from build123d import *

# Parameters (mm, degrees)
BOSS_EXTRUDE1_DEPTH = 9.525
CUT_EXTRUDE11_DEPTH = 109.249530891
CUT_EXTRUDE12_DEPTH = 109.249530891
CUT_EXTRUDE1_DEPTH  = 164.459241155
FILLET25_R          = 0.79375
CUT_EXTRUDE8_DEPTH  = 7.112
FILLET31_R          = 0.79375
FILLET32_R          = 0.5
DELETEFACE2_START   = 2.413
DELETEFACE2_DEPTH   = 8.587
DELETEFACE2_2_DEPTH = 9.525
DELETEFACE3_START   = 2.413
DELETEFACE3_DEPTH   = 7.112
SKETCH42_R          = 2
CUT_EXTRUDE13_DEPTH = 1


with BuildPart() as part:
    # Sketch2 → Boss-Extrude1 (new body)
    with BuildSketch(Plane(origin=(0, 0, 0), x_dir=(1, 0, 0), z_dir=(0, 1, 0))):
        Polygon((95.501036211, 33.603610094), (107.801036211, 122.503610094), (-44.198963789, 122.503610094), (19.301036211, 33.603610094), align=None)
    extrude(amount=BOSS_EXTRUDE1_DEPTH)

    # Sketch40 → Cut-Extrude11 (cut, along a direction that is not the sketch's normal)
    with BuildSketch(Plane(origin=(0, 0, -122.503610094), x_dir=(-1, 0, 0), z_dir=(0, 0, -1))):
        Polygon((44.198963789, 4.7625), (25.464097027, 0), (44.198963789, 0), align=None)
    extrude(amount=-CUT_EXTRUDE11_DEPTH, dir=(-0.5812381937190961, 0, -0.8137334712067352), mode=Mode.SUBTRACT)

    # Sketch41 → Cut-Extrude12 (cut, along a direction that is not the sketch's normal)
    with BuildSketch(Plane(origin=(0, 0, -122.503610094), x_dir=(-1, 0, 0), z_dir=(0, 0, -1))):
        Polygon((44.198963789, 4.7625), (44.198963789, 9.525), (25.464097027, 9.525), align=None)
    extrude(amount=-CUT_EXTRUDE12_DEPTH, dir=(-0.5812381937190961, 0, -0.8137334712067352), mode=Mode.SUBTRACT)

    # Sketch3 → Cut-Extrude1 (cut, through all)
    with BuildSketch(Plane(origin=(0, 9.525, 0), x_dir=(1, 0, 0), z_dir=(0, 1, 0))):
        Polygon((96.991616373, 44.376990288), (78.121375316, 46.987833539), (81.602499651, 72.148154947), (100.472740707, 69.537311696), align=None)
    extrude(amount=-CUT_EXTRUDE1_DEPTH, mode=Mode.SUBTRACT)

    # Fillet25
    fillet25_edges = [part.edges().sort_by_distance(p)[0] for p in [
        (100.472740707, 4.7625, -69.537311696),
        (96.991616373, 4.7625, -44.376990288),
        (78.121375316, 4.7625, -46.987833539),
        (81.602499651, 4.7625, -72.148154947),
    ]]
    fillet(fillet25_edges, radius=FILLET25_R)

    # Sketch4 → Cut-Extrude8 (cut)
    with BuildSketch(Plane(origin=(0, 9.525, 0), x_dir=(1, 0, 0), z_dir=(0, 1, 0))):
        with BuildLine():
            Line((91.432981633, 84.938583056), (91.87398018, 88.3325177))
            ThreePointArc((91.87398018, 88.3325177), (91.880119161, 88.935768076), (91.743819438, 89.523450889))
            Line((91.743819438, 89.523450889), (84.365995583, 109.929022071))
            ThreePointArc((84.365995583, 109.929022071), (84.052194516, 110.530485922), (83.590381446, 111.027435178))
            Line((83.590381446, 111.027435178), (69.63117281, 122.503610094))
            Line((69.63117281, 122.503610094), (65.631546235, 122.503610094))
            Line((65.631546235, 122.503610094), (81.977330858, 109.065378145))
            Line((81.977330858, 109.065378145), (88.524922018, 90.956062972))
            ThreePointArc((88.524922018, 90.956062972), (86.871368444, 87.055321455), (82.635738177, 86.958058718))
            ThreePointArc((82.635738177, 86.958058718), (82.108570303, 87.435753172), (81.573856943, 87.904986143))
            ThreePointArc((81.573856943, 87.904986143), (80.279037974, 88.75135311), (78.792534366, 89.179372068))
            Line((78.792534366, 89.179372068), (71.259162002, 90.172380139))
            Line((71.259162002, 90.172380139), (70.399965305, 83.95114873))
            Line((70.399965305, 83.95114873), (68.995626594, 73.78267842))
            Line((68.995626594, 73.78267842), (81.599351809, 72.105893611))
            Line((81.599351809, 72.105893611), (81.450209567, 70.968016338))
            Line((81.450209567, 70.968016338), (82.559812791, 70.82309653))
            Line((82.559812791, 70.82309653), (82.351161676, 69.22552369))
            Line((82.351161676, 69.22552369), (86.280730255, 68.712302106))
            Line((86.280730255, 68.712302106), (86.63642856, 71.435766832))
            Line((86.63642856, 71.435766832), (89.626769646, 71.037935364))
            Line((89.626769646, 71.037935364), (91.432981633, 84.938583056))
        make_face()
    extrude(amount=-CUT_EXTRUDE8_DEPTH, mode=Mode.SUBTRACT)

    # Fillet31
    # the kernel refuses this fillet: 0.79375 mm, written as the material it adds along each edge
    with BuildSketch(Plane(origin=(71.259162002, 9.525, -90.172380139), x_dir=(0.9914240578116118, 0, 0.13068411377194142), z_dir=(0, -1, 0))) as fillet31_piece_1:
        with BuildLine():
            CenterArc((FILLET31_R * 0.993838975456, FILLET31_R), FILLET31_R, 180.35409036, 89.64590964)
            Line((-FILLET31_R * 0.00614192814136, FILLET31_R * 0.993819996707), (0, 0))
            Line((0, 0), (FILLET31_R * 0.993838975456, 0))
        make_face()
    extrude(amount=9.084149217)
    with BuildSketch(Plane(origin=(68.995626594, 9.525, -73.78267842), x_dir=(0.13680862211806724, 0, -0.9905974969250406), z_dir=(0, -1, 0))) as fillet31_piece_2:
        with BuildLine():
            CenterArc((FILLET31_R * 1.00498928997, FILLET31_R), FILLET31_R, 179.714846688, 90.285153312)
            Line((FILLET31_R * 0.00500167453449, FILLET31_R * 1.00497684362), (0, 0))
            Line((0, 0), (FILLET31_R * 1.00498928997, 0))
        make_face()
    extrude(amount=9.106275622)
    # the kernel refuses this fillet: 0.79375 mm, written as the material it takes off along each edge
    with BuildSketch(Plane(origin=(89.626769646, 11.493028645, -71.037935364), x_dir=(0.9905638349724125, 0, 0.13705213914692133), z_dir=(0, -1, 0))) as fillet31_2_piece_1:
        with BuildLine():
            CenterArc((FILLET31_R * 0.991762466743, -FILLET31_R), FILLET31_R, 90, 89.526074815)
            Line((-FILLET31_R * 0.00820332414174, -FILLET31_R * 0.991728539427), (0, 0))
            Line((0, 0), (FILLET31_R * 0.991762466743, 0))
        make_face()
    extrude(amount=9.080028645, mode=Mode.SUBTRACT)
    with BuildSketch(Plane(origin=(81.599351809, 11.470712134, -72.105893611), x_dir=(-0.99126610392599, 0, -0.1318768789719729), z_dir=(0, -1, 0))) as fillet31_2_piece_2:
        with BuildLine():
            CenterArc((0.778284853, -0.79375), FILLET31_R, 90, 79.138737607)
            Line((-0.001246175, -0.644182498), (0, 0))
            Line((0, 0), (0.778284853, 0))
        make_face()
    extrude(amount=9.057712134, mode=Mode.SUBTRACT)

    # Fillet32
    fillet32_edges = [part.edges().sort_by_distance(p)[0] for p in [
        (-12.448963789, 4.7625, -78.053610094),
    ]]
    fillet(fillet32_edges, radius=FILLET32_R)

    # DeleteFace2: read off the stored shape, not the designer's step
    # DeleteFace2 outline → DeleteFace2 (cut)
    with BuildSketch(Plane(origin=(0, 0, 0), x_dir=(1, 0, 0), z_dir=(0, 1, 0)).offset(DELETEFACE2_START)):
        with BuildLine():
            Line((71.259162002, 90.172380139), (71.151239195, 89.390937708))
            ThreePointArc((71.151239195, 89.390937708), (71.456370289, 89.91363683), (72.041256474, 90.06928871))
            Line((72.041256474, 90.06928871), (71.259162002, 90.172380139))
        make_face()
        with BuildLine():
            Line((68.995626594, 73.78267842), (69.786369725, 73.677478882))
            ThreePointArc((69.786369725, 73.677478882), (69.259466687, 73.983520547), (69.104760234, 74.572888196))
            Line((69.104760234, 74.572888196), (68.995626594, 73.78267842))
        make_face()
    extrude(amount=DELETEFACE2_DEPTH, mode=Mode.SUBTRACT)

    # DeleteFace2 2 outline → DeleteFace2 2 (add)
    with BuildSketch(Plane(origin=(0, 0, 0), x_dir=(1, 0, 0), z_dir=(0, 1, 0))):
        with BuildLine():
            ThreePointArc((80.827864414, 72.208531388), (81.305090173, 71.961554565), (81.515634323, 71.467172994))
            ThreePointArc((81.515634323, 71.467172994), (81.745680073, 71.840109312), (82.138550491, 72.034159252))
            Line((82.138550491, 72.034159252), (80.827864414, 72.208531388))
        make_face()
    extrude(amount=DELETEFACE2_2_DEPTH)

    # DeleteFace3: read off the stored shape, not the designer's step
    # DeleteFace3 outline → DeleteFace3 (add)
    with BuildSketch(Plane(origin=(0, 0, 0), x_dir=(1, 0, 0), z_dir=(0, 1, 0)).offset(DELETEFACE3_START)):
        with BuildLine():
            Line((82.388759695, 72.039369812), (90.406552846, 70.93004635))
            ThreePointArc((90.406552846, 70.93004635), (89.884432105, 71.234645894), (89.728205023, 71.818584289))
            Line((89.728205023, 71.818584289), (91.87398018, 88.3325177))
            ThreePointArc((91.87398018, 88.3325177), (91.880119161, 88.935768076), (91.743819438, 89.523450889))
            Line((91.743819438, 89.523450889), (84.365995583, 109.929022071))
            ThreePointArc((84.365995583, 109.929022071), (84.052194516, 110.530485922), (83.590381446, 111.027435178))
            Line((83.590381446, 111.027435178), (69.63117281, 122.503610094))
            Line((69.63117281, 122.503610094), (65.631546235, 122.503610094))
            Line((65.631546235, 122.503610094), (81.977330858, 109.065378145))
            Line((81.977330858, 109.065378145), (88.524922018, 90.956062972))
            ThreePointArc((88.524922018, 90.956062972), (86.871368444, 87.055321455), (82.635738177, 86.958058718))
            ThreePointArc((82.635738177, 86.958058718), (82.108570303, 87.435753172), (81.573856943, 87.904986143))
            ThreePointArc((81.573856943, 87.904986143), (80.279037974, 88.75135311), (78.792534366, 89.179372068))
            Line((78.792534366, 89.179372068), (71.259162002, 90.172380139))
            Line((71.259162002, 90.172380139), (68.995626594, 73.78267842))
            Line((68.995626594, 73.78267842), (82.138550491, 72.034159252))
            ThreePointArc((82.138550491, 72.034159252), (82.263448445, 72.04668771), (82.388759695, 72.039369812))
        make_face()
    extrude(amount=DELETEFACE3_DEPTH)

    # Sketch42 → Cut-Extrude13 (cut)
    with BuildSketch(Plane(origin=(11.327516936, 0, -81.871240295), x_dir=(0.9905638349724135, 0, 0.13705213914691416), z_dir=(-0.13705213914691416, 0, 0.9905638349724135))):
        with Locations((73.988256108, 4.7625)):
            Circle(SKETCH42_R)
    extrude(amount=-CUT_EXTRUDE13_DEPTH, mode=Mode.SUBTRACT)


solid = part.part
Input: part model. Units: mm. Frame: model coordinates. A direction names the side the tool comes from. Give positions to 0.01 mm unless a question says otherwise; leave off trailing zeros. Write each loop counter-clockwise with the first axis right and the second up, starting at its lowest first coordinate (ties: lowest second). Pieces come first, ordered by that corner, then holes. Notation, with made-up numbers: M 1.5,60.25 L 44.5,60.25 A10 ccw 44.5,74.25 Z; hole C 79.25,77 d5. An arc over 180 degrees is marked long. Use one line per item in the form item = value.
1. Mould query, pull axis X, two halves, no side actions, for faces 1 (the face through (86.515, 3.996, -71.966)), 2 (the face through (84.727, 4.791, -72.725)), 3 (the face through (-2.47, 1.59, -81.55)), 4 (the face through (58, 5, -33.604)). Classes: released by +X, released by -X, zero draft, split by the parting line, or undercut.
Outcome:
face_1 = undercut
face_2 = undercut
face_3 = released by -X
face_4 = zero draft
2. Ray query, L1, parallel to X at y = 5, z = -107.5; L2, parallel to Z at x = 98, y = 3.5; L3, parallel to X at y = 4.5, z = -82. Return the intervals inside material, ascending.
Outcome:
L1 = -31.96 to 105.73
L2 = -122.5 to -69.88
L3 = -13.73 to 102.2
3. First-contact query: P1, Ø1.5, axis at y = 4, z = -106, coming from the +X side; P2, Ø1.5, axis at y = 4, z = -56, coming from the +X side; P3, Ø5, axis at y = 2, z = -112, coming from the -X side. Flat tips, straight axial feed; report the tip coordinate or a pass-through.
Outcome:
P1 = 105.62
P2 = 79.47
P3 = -35.59
4. Cut plane A-A on x = 25. Return loops of the section in (y, z) (3 decimals), and give its area (3 significant figures).
Outcome:
outline = M 0,-122.504 L 9.525,-122.504 L 9.525,-51.854 L 6.211,-33.604 L 3.314,-33.604 L 0,-51.854 Z
area = 786 mm²
5. Reachability of faces 5 (the face through (-10.5, 4.77, -77.35)), 6 (the face through (87.678, 4.829, -45.666)) from +Z, -Z, +X, -X, +Y, -Y: full face, straight path, thin tool, end or side. Return the list, or none.
Outcome:
face_5 = +Z, -X
face_6 = +X, +Y, -Y
